```python
from build123d import *

# Parameters (mm, degrees)
EXTRUDE_1_DEPTH     = 100
SHELL_1_T           = -20
CUT_EXTRUDE_1_DEPTH = 50
SKETCH_3_R          = 60
CUT_EXTRUDE_2_DEPTH = 50
SKETCH_5_R          = 60
SKETCH_5_R_2        = 40
EXTRUDE_2_DEPTH     = 20


with BuildPart() as part:
    # 草图1 → 凸台-拉伸1 (new body)
    with BuildSketch(Plane.XY):
        with BuildLine():
            Line((3, 0), (497, 0))
            ThreePointArc((497, 0), (499.121320344, -0.878679656), (500, -3))
            Line((500, -3), (500, -567))
            ThreePointArc((500, -567), (499.121320344, -569.121320344), (497, -570))
            Line((497, -570), (3, -570))
            ThreePointArc((3, -570), (0.878679656, -569.121320344), (0, -567))
            Line((0, -567), (0, -3))
            ThreePointArc((0, -3), (0.878679656, -0.878679656), (3, 0))
        make_face()
    extrude(amount=EXTRUDE_1_DEPTH)

    # 抽壳1
    shell_1_openings = [part.faces().sort_by_distance(p)[0] for p in [
        (250, -285, 100),
    ]]
    offset(amount=SHELL_1_T, openings=shell_1_openings, kind=Kind.INTERSECTION)

    # 草图2 → 切除-拉伸1 (cut)
    with BuildSketch(Plane.XY.offset(100)):
        Polygon((4.785, -5.49), (495.215, -5.49), (495.215, -20), (495.215, -550), (495.215, -564.51), (4.785, -564.51), (4.785, -550), (4.785, -20), align=None)
    extrude(amount=-CUT_EXTRUDE_1_DEPTH, mode=Mode.SUBTRACT)

    # 草图3 → 切除-拉伸2 (cut)
    with BuildSketch(Plane(origin=(0, 0, 0), x_dir=(-1, 0, 0), z_dir=(0, 0, -1))):
        with Locations((-250, -150)):
            Circle(SKETCH_3_R)
    extrude(amount=-CUT_EXTRUDE_2_DEPTH, mode=Mode.SUBTRACT)

    # 草图5 → 凸台-拉伸2 (add)
    with BuildSketch(Plane(origin=(0, 0, 0), x_dir=(-1, 0, 0), z_dir=(0, 0, -1))):
        with Locations((-250, -150)):
            Circle(SKETCH_5_R)
        with Locations((-250, -150)):
            Circle(SKETCH_5_R_2, mode=Mode.SUBTRACT)
    extrude(amount=-EXTRUDE_2_DEPTH)


solid = part.part
```
For this review, take the finished solid that the model builds, in its own axes (mm). A direction names the side the tool comes from. Coordinates: 2 decimals unless noted, no trailing zeros. Write each loop counter-clockwise with the first axis right and the second up, starting at its lowest first coordinate (ties: lowest second). Pieces come first, ordered by that corner, then holes. Notation, with made-up numbers: (-13, -16.75) - (18, -16.75) arc R19 ccw to (18, 16.25) - close; hole circle Ø11 at (35, 49.5). An arc over 180 degrees is marked (long way). Answer in a Markdown table with one row per item. Add a question column.
Q1. Draft analysis for pull direction X (two halves, no side actions). For faces 3 (the flat face through (0, -289, 49)), 4 (the flat face through (480, -281, 35)), 5 (the flat face through (253, -281, 20)), 6 (the flat face through (500, -281, 49)), state which applies: +X half, -X half, draft (parallel to the pull), parting line (faces both ways), or undercut.
Q2. We need section D-D, the plane y = -304.5. State the section outline as (x, z) points (3 decimals).
Q3. Tool access review of faces 1 (the flat face through (487, -284, 50)), 2 (the flat face through (247, 0, 49)): name each direction out of +Z, -Z, +X, -X, +Y, -Y from which nothing blocks a thin tool from reaching the whole face with its end or side.
Q4. We need section B-B, the plane y = -150. State the section outline as (x, z) points (3 decimals), and give its area (3 significant figures).
Q5. For P1, Ø3, axis at x = 357, y = -314.5, coming from the +Z side, flat-tipped, find the tip position at first contact; note if it passes through.
Q6. For probe 1 along Y at (x, z) = (193, 70.5); probe 2 along Y at (x, z) = (250, 7.75); probe 3 along X at (y, z) = (-90, 58.5) (3 decimals), list the stretches that pass through material, from the lowest coordinate up.
Q7. We need section A-A, the plane x = 250. State the section outline as (y, z) points.
Q8. We need section C-C, the plane z = 33. State the section outline as (x, y) points.
Answer list:
| question | item | result |
|---|---|---|
| 1 | face 3 | -X half |
| 1 | face 4 | undercut |
| 1 | face 5 | undercut |
| 1 | face 6 | +X half |
| 2 | outline | (0, 0) - (500, 0) - (500, 100) - (495.215, 100) - (495.215, 50) - (480, 50) - (480, 20) - (20, 20) - (20, 50) - (4.785, 50) - (4.785, 100) - (0, 100) - close |
| 3 | face 1 | +Z |
| 3 | face 2 | +Z, -Z, +X, -X, +Y |
| 4 | outline | (0, 0) - (210, 0) - (210, 20) - (20, 20) - (20, 50) - (4.785, 50) - (4.785, 100) - (0, 100) - close; (290, 0) - (500, 0) - (500, 100) - (495.215, 100) - (495.215, 50) - (480, 50) - (480, 20) - (290, 20) - close |
| 4 | area | 10,100 mm2 |
| 5 | P1 | stops at z = 20 |
| 6 | probe 1 | y = -570 to -564.51, -5.49 to 0 |
| 6 | probe 2 | y = -570 to -190, -110 to 0 |
| 6 | probe 3 | x = 0 to 4.785, 495.215 to 500 |
| 7 | outline | (-570, 0) - (-190, 0) - (-190, 20) - (-550, 20) - (-550, 50) - (-564.51, 50) - (-564.51, 100) - (-570, 100) - close; (-110, 0) - (0, 0) - (0, 100) - (-5.49, 100) - (-5.49, 50) - (-20, 50) - (-20, 20) - (-110, 20) - close |
| 8 | outline | (0, -567) arc R3 ccw to (3, -570) - (497, -570) arc R3 ccw to (500, -567) - (500, -3) arc R3 ccw to (497, 0) - (3, 0) arc R3 ccw to (0, -3) - close; hole (20, -550) - (480, -550) - (480, -20) - (20, -20) - close |
